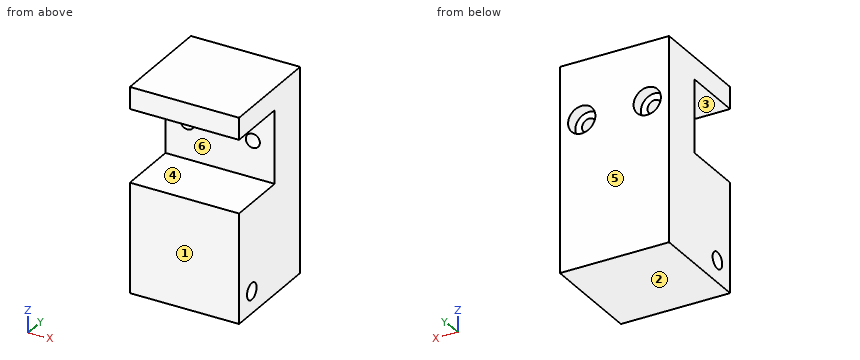
from build123d import *

# Parameters (mm, degrees)
BOSS_EXTRUDE1_DEPTH                            = 19.05
CBORE_FOR_2_SOCKET_HEAD_CAP_SCREW1_D           = 2.4384
CBORE_FOR_2_SOCKET_HEAD_CAP_SCREW1_CBORE_D     = 4.7625
CBORE_FOR_2_SOCKET_HEAD_CAP_SCREW1_CBORE_DEPTH = 2.1844
F_6_40_TAPPED_HOLE2_D                          = 2.8702


with BuildPart() as part:
    # Sketch1 → Boss-Extrude1 (new body)
    with BuildSketch(Plane(origin=(0, 0, 0), x_dir=(0, 0, -1), z_dir=(1, 0, 0))):
        Polygon((-8.89, 0), (10.16, 0), (10.16, 18.288), (-25.4, 18.288), (-25.4, 0), (-21.59, 0), (-21.59, 10.668), (-8.89, 10.668), align=None)
    extrude(amount=BOSS_EXTRUDE1_DEPTH)

    # CBORE for #2 Socket Head Cap Screw1 (through all)
    with Locations(Plane(origin=(0, 18.288, 0), x_dir=(-1, 0, 0), z_dir=(0, 1, 0))):
        with Locations((-3.81, 15.24), (-15.24, 15.24)):
            CounterBoreHole(CBORE_FOR_2_SOCKET_HEAD_CAP_SCREW1_D / 2, CBORE_FOR_2_SOCKET_HEAD_CAP_SCREW1_CBORE_D / 2, CBORE_FOR_2_SOCKET_HEAD_CAP_SCREW1_CBORE_DEPTH)

    # #6-40 Tapped Hole2 (through all)
    with Locations(Plane.ZY):
        with Locations((-6.35, 3.81)):
            Hole(F_6_40_TAPPED_HOLE2_D / 2)


solid = part.part
Geometry check sheet. Reference: the model listing, model coordinates, mm. Face numbers are marked on the shaded views. A direction names the side the tool comes from. Give positions to 0.01 mm unless a question says otherwise; leave off trailing zeros. Loops run counter-clockwise (first coordinate to the right, second up) from the corner with the lowest first, then second, coordinate; pieces in that order, holes last. Notation, with made-up numbers: (31, -33) -> (61, -33) arc R34 cw to (61, 3) -> close; hole circle Ø10 at (-24.5, -3.75). An arc over 180 degrees is marked (long way). Answer in a Markdown table with one row per item. Add a question column.
1) Gauge pin test, flat ends, axial feed: P1, Ø10, axis at x = 12.5, z = 14.5, coming from the -Y side; P2, Ø4, axis at x = 15.24, z = 15.24, coming from the +Y side; P3, Ø6, axis at y = 7, z = 14.5, coming from the +X side. Record the tip position at first contact, or that the pin passes through.
2) Set-up check for the marked faces 5 and 6: record each of +Z, -Z, +X, -X, +Y, -Y from which the full face is reachable in a straight line by a thin tool's end or side.
3) Cross-section at B-B on z = 15.24. Record the boundary of the cut face in (x, y), and give its area (3 significant figures).
4) Draft check along Z on the marked faces 1, 2, 3 and 4. Enter one of: pulls with the +Z half, pulls with the -Z half, needs draft (parallel to the pull), parting line crosses it, or undercut.
5) Cross-section at A-A on x = 3.81. Record the boundary of the cut face in (y, z).
6) Cross-section at D-D on z = -6.35. Record the boundary of the cut face in (x, y).
7) Material ranges on probe 1 along Z at (x, y) = (1.5, 6.5); probe 2 along Y at (x, z) = (9.5, -6.35); probe 3 along Z at (x, y) = (3.81, 13.25), recorded low to high. Write a range as from..to.
8) Cross-section at C-C on y = 8.75. Record the boundary of the cut face in (x, z).
Outcome:
| question | item | result |
|---|---|---|
| 1 | P1 | stops at y = 10.67 |
| 1 | P2 | stops at y = 16.1 |
| 1 | P3 | passes through |
| 2 | face 5 | +Z, -Z, +X, -X, +Y |
| 2 | face 6 | +X, -X, -Y |
| 3 | outline | (0, 10.67) -> (2.59, 10.67) -> (2.59, 16.1) -> (1.43, 16.1) -> (1.43, 18.29) -> (0, 18.29) -> close; (5.03, 10.67) -> (14.02, 10.67) -> (14.02, 16.1) -> (12.86, 16.1) -> (12.86, 18.29) -> (6.19, 18.29) -> (6.19, 16.1) -> (5.03, 16.1) -> close; (16.46, 10.67) -> (19.05, 10.67) -> (19.05, 18.29) -> (17.62, 18.29) -> (17.62, 16.1) -> (16.46, 16.1) -> close |
| 3 | area | 97.8 mm^2 |
| 4 | face 1 | needs draft |
| 4 | face 2 | pulls with the -Z half |
| 4 | face 3 | undercut |
| 4 | face 4 | undercut |
| 5 | outline | (0, -10.16) -> (18.29, -10.16) -> (18.29, 12.86) -> (16.1, 12.86) -> (16.1, 14.02) -> (10.67, 14.02) -> (10.67, 8.89) -> (0, 8.89) -> close; (0, 21.59) -> (10.67, 21.59) -> (10.67, 16.46) -> (16.1, 16.46) -> (16.1, 17.62) -> (18.29, 17.62) -> (18.29, 25.4) -> (0, 25.4) -> close; hole circle Ø2.87 at (3.81, -6.35) |
| 6 | outline | (0, 0) -> (19.05, 0) -> (19.05, 2.37) -> (0, 2.37) -> close; (0, 5.25) -> (19.05, 5.25) -> (19.05, 18.29) -> (0, 18.29) -> close |
| 7 | probe 1 | z = -10.16..8.89, 21.59..25.4 |
| 7 | probe 2 | y = 0..2.37, 5.25..18.29 |
| 7 | probe 3 | z = -10.16..14.02, 16.46..25.4 |
| 8 | outline | (0, -10.16) -> (19.05, -10.16) -> (19.05, 8.89) -> (0, 8.89) -> close; (0, 21.59) -> (19.05, 21.59) -> (19.05, 25.4) -> (0, 25.4) -> close |
